```python
from build123d import *

# Parameters (mm, degrees)
EXTRUDE_1_DEPTH          = 40
EXTRUDE_1_DEPTH_BACK     = 40
CUT_EXTRUDE_1_DEPTH      = 30
CUT_EXTRUDE_1_DEPTH_BACK = 30
SKETCH_2_R               = 40
SKETCH_3_R               = 15
CUT_EXTRUDE_2_DEPTH      = 75
SKETCH_4_W               = 67.943944805
SKETCH_4_H               = 80
EXTRUDE_2_DEPTH          = 19
SKETCH_5_W               = 10.069063792
SKETCH_5_H               = 80
EXTRUDE_3_DEPTH          = 19
SKETCH_6_R               = 8.162997033
CUT_EXTRUDE_3_DEPTH      = 34


with BuildPart() as part:
    # Sketch 1 → Extrude 1 (new, two sides: drawn at the far end of the back side and taken through both)
    with BuildSketch(Plane.XY.offset(-EXTRUDE_1_DEPTH_BACK)):
        with BuildLine():
            Line((-60, 0), (-35, 0))
            ThreePointArc((-35, 0), (0, -35), (35, 0))
            Line((35, 0), (60, 0))
            ThreePointArc((60, 0), (0, -60), (-60, 0))
        make_face()
    extrude(amount=EXTRUDE_1_DEPTH + EXTRUDE_1_DEPTH_BACK)

    # Sketch 2 → Cut-Extrude 1 (cut, two sides: drawn at the far end of the back side and taken through both)
    with BuildSketch(Plane.XY.offset(-CUT_EXTRUDE_1_DEPTH_BACK)):
        Circle(SKETCH_2_R)
    extrude(amount=CUT_EXTRUDE_1_DEPTH + CUT_EXTRUDE_1_DEPTH_BACK, mode=Mode.SUBTRACT)

    # Sketch 3 → Cut-Extrude 2 (cut)
    with BuildSketch(Plane(origin=(0, 0, 0), x_dir=(1, 0, 0), z_dir=(0, 1, 0))):
        with Locations(Location((0, 0, 0), (0, 0, 270))):
            Circle(SKETCH_3_R)
    extrude(amount=-CUT_EXTRUDE_2_DEPTH, mode=Mode.SUBTRACT)

    # Sketch 4 → Extrude 2 (add)
    with BuildSketch(Plane(origin=(0, 0, 0), x_dir=(1, 0, 0), z_dir=(0, 1, 0))):
        with Locations((74.586023034, 0)):
            Rectangle(SKETCH_4_W, SKETCH_4_H)
    extrude(amount=-EXTRUDE_2_DEPTH)

    # Sketch 5 → Extrude 3 (add)
    with BuildSketch(Plane(origin=(0, 0, 0), x_dir=(1, 0, 0), z_dir=(0, 1, 0))):
        with Locations((103.52346354, 0)):
            Rectangle(SKETCH_5_W, SKETCH_5_H)
    extrude(amount=EXTRUDE_3_DEPTH)

    # Sketch 6 → Cut-Extrude 3 (cut)
    with BuildSketch(Plane(origin=(0, 0, 0), x_dir=(1, 0, 0), z_dir=(0, 1, 0))):
        with Locations(Location((71.232555132, 0, 0), (0, 0, 270))):
            Circle(SKETCH_6_R)
    extrude(amount=-CUT_EXTRUDE_3_DEPTH, mode=Mode.SUBTRACT)


solid = part.part
```
Work out the finished part from the listing and answer in its coordinate system (mm). A direction names the side the tool comes from. Give positions to 0.01 mm unless a question says otherwise; leave off trailing zeros. Loops run counter-clockwise (first coordinate to the right, second up) from the corner with the lowest first, then second, coordinate; pieces in that order, holes last. Notation, with made-up numbers: (-36, 8.5) -> (-12, 8.5) arc R32 cw to (-12, 35.5) -> close; hole circle Ø11 at (49.25, 47.5). An arc over 180 degrees is marked (long way). Use CSV: the item, a comma, the result in double quotes.
1. The part is cut by section C-C (z = 0). Write down the section's boundary in (x, y), then the cut area to 3 significant figures.
Found:
outline,"(-60, 0) arc R60 ccw to (-15, -58.09) -> (-15, -37.08) arc R40 cw to (-40, 0) -> close; (15, -58.09) arc R60 ccw to (56.91, -19) -> (63.07, -19) -> (63.07, 0) -> (40, 0) arc R40 cw to (15, -37.08) -> close; (79.4, -19) -> (108.56, -19) -> (108.56, 19) -> (98.49, 19) -> (98.49, 0) -> (79.4, 0) -> close"
area,"3,350 mm^2"
2. The part is cut by section A-A (y = -5.5). Write down the section's boundary in (x, z), then the cut area to 3 significant figures.
Found:
outline,"(-59.75, -40) -> (-34.57, -40) -> (-34.57, -30) -> (-39.62, -30) -> (-39.62, 30) -> (-34.57, 30) -> (-34.57, 40) -> (-59.75, 40) -> close; (34.57, -40) -> (108.56, -40) -> (108.56, 40) -> (34.57, 40) -> (34.57, 30) -> (39.62, 30) -> (39.62, -30) -> (34.57, -30) -> close; hole circle Ø16.33 at (71.23, 0)"
area,"7,120 mm^2"
3. The part is cut by section D-D (z = 20). Write down the section's boundary in (x, y), then the cut area to 3 significant figures.
Found:
outline,"(-60, 0) arc R60 ccw to (56.91, -19) -> (108.56, -19) -> (108.56, 19) -> (98.49, 19) -> (98.49, 0) -> (40, 0) arc R40 cw to (-40, 0) -> close"
area,"4,270 mm^2"
4. The part is cut by section B-B (x = 0). Write down the section's boundary in (y, z).
Found:
outline,"(-60, -40) -> (-35, -40) -> (-35, -30) -> (-40, -30) -> (-40, -15) -> (-60, -15) -> close; (-60, 15) -> (-40, 15) -> (-40, 30) -> (-35, 30) -> (-35, 40) -> (-60, 40) -> close"
5. Straight lines are drawn through the part: line 1 (Z direction, x = -10, y = -35); line 2 (Z direction, x = 0, y = -47.25); line 3 (X direction, y = -5.25, z = 0). For each, find the intervals that lie inside material, in ascending order.
Found:
line 1,"-40 to -30, 30 to 40"
line 2,"-40 to -15, 15 to 40"
line 3,"-59.77 to -39.65, 39.65 to 63.07, 79.4 to 108.56"
6. A tool of negligible diameter and unlimited length cuts with its end or side. For faces 1 (the flat face through (66, 0, -9)), 2 (the flat face through (82, -19, -1)), 3 (the flat face through (6, -35, -30)), from which of +Z, -Z, +X, -X, +Y, -Y can it reach the whole face along a straight path? Write none if from no direction.
Found:
face 1,"+Z, -Z, -X, +Y"
face 2,"+Z, -Z, +X, -Y"
face 3,"+Y"
7. Flat-ended cylindrical pins translate along their axes: pin 1 Ø8 at (x, z) = (-1, 29) entering from +Y; pin 2 Ø1.5 at (y, z) = (-31.5, 22.5) entering from +X; pin 3 Ø6 at (y, z) = (-31.5, 5) entering from +X. Find the tip coordinate at first contact, or state that the pin passes through.
Found:
pin 1,"y = -34.66"
pin 2,"x = 51.52"
pin 3,"x = 52.8"
8. The mould has two halves that part along X. Classify faces 4 (the cylindrical face through (12.65, -48.39, 8.06)), 5 (the flat face through (98.489, 9, 1)), 6 (the flat face through (24, -27, 40)): +X half, -X half, draft (parallel to the pull), parting line (faces both ways), or undercut.
Found:
face 4,"undercut"
face 5,"-X half"
face 6,"draft"
